from build123d import *

# Parameters (mm, degrees)
SKETCH1_W           = 20
SKETCH1_H           = 20
BOSS_EXTRUDE1_DEPTH = 279.4
SKETCH3_R           = 7.5
BOSS_EXTRUDE2_DEPTH = 1.5
CUT_EXTRUDE1_DEPTH  = 266.7


with BuildPart() as part:
    # Sketch1 → Boss-Extrude1 (new body)
    with BuildSketch(Plane(origin=(0, 0, 0), x_dir=(0, 0, -1), z_dir=(1, 0, 0))):
        with Locations((-10, 10)):
            Rectangle(SKETCH1_W, SKETCH1_H)
    extrude(amount=BOSS_EXTRUDE1_DEPTH)

    # Sketch3 → Boss-Extrude2 (add)
    with BuildSketch(Plane(origin=(0, 0, 0), x_dir=(-1, 0, 0), z_dir=(0, 0, -1))):
        with Locations(Location((-10, 10, 0), (0, 0, 180))):
            Circle(SKETCH3_R)
    extrude(amount=BOSS_EXTRUDE2_DEPTH)

    # Sketch2 → Cut-Extrude1 (cut)
    with BuildSketch(Plane(origin=(279.4, 0, 0), x_dir=(0, 0, -1), z_dir=(1, 0, 0))):
        with BuildLine():
            ThreePointArc((-2.5, 10), (-3.070903506, 12.870125743), (-4.696699141, 15.303300859))
            Line((-4.696699141, 15.303300859), (-15.303300859, 4.696699141))
            ThreePointArc((-15.303300859, 4.696699141), (-7.129874257, 3.070903506), (-2.5, 10))
        make_face()
        with BuildLine():
            Line((-15.303300859, 4.696699141), (-4.696699141, 15.303300859))
            ThreePointArc((-4.696699141, 15.303300859), (-15.303300859, 15.303300859), (-15.303300859, 4.696699141))
        make_face()
    extrude(amount=-CUT_EXTRUDE1_DEPTH, mode=Mode.SUBTRACT)


solid = part.part
Input: part model. Units: mm. Frame: model coordinates. Coordinates: 2 decimals unless noted, no trailing zeros. Loops run counter-clockwise (first coordinate to the right, second up) from the corner with the lowest first, then second, coordinate; pieces in that order, holes last.
(1) Material intervals for probe 1 along Y at (x, z) = (198.5, 10.5); probe 2 along Z at (x, y) = (189.5, 9.75); probe 3 along Y at (x, z) = (88.5, 16.5), sorted ascending.
(2) First-contact query: pin 1 Ø7.5 at (y, z) = (8.5, 10) entering from +X; pin 2 Ø5 at (x, y) = (69, 6.5) entering from -Z. Flat tips, straight axial feed; report the tip coordinate or a pass-through.
(3) Pull-direction query (Y, two-part tool) for faces 1 (the face through (8.37, 17.32, -0.74)), 2 (the face through (138, 10, 0)), 3 (the face through (12.7, 10, 10)), 4 (the face through (138, 20, 10)); classes: released by +Y, released by -Y, zero draft, split by the parting line, or undercut.
(4) Section C-C on x = 10. Return the cut outline in (y, z).
(5) Section B-B on x = 247.5. Return the cut outline in (y, z), then the cut area to 3 significant figures.
(6) Section A-A on z = 10. Return the cut outline in (x, y).
Data:
1. probe 1: y = 0 to 2.52, 17.48 to 20
1. probe 2: z = 0 to 2.5, 17.5 to 20
1. probe 3: y = 0 to 6.26, 13.74 to 20
2. pin 1: stops at x = 12.7
2. pin 2: stops at z = 0
3. face 1: split by the parting line
3. face 2: zero draft
3. face 3: undercut
3. face 4: released by +Y
4. outline: (0, 0) - (2.5, 0) - (2.5, -1.5) - (17.5, -1.5) - (17.5, 0) - (20, 0) - (20, 20) - (0, 20) - close
5. outline: (0, 0) - (20, 0) - (20, 20) - (0, 20) - close; hole circle Ø15 at (10, 10)
5. area: 223 mm2
6. outline: (0, 0) - (279.4, 0) - (279.4, 2.5) - (12.7, 2.5) - (12.7, 17.5) - (279.4, 17.5) - (279.4, 20) - (0, 20) - close
